Autodesk Inventor part; units mm, degrees
ref_plane "Work Plane2" through (26.9102, -85.3653, -23.8679) normal (0, 0, -1) x (0, 1, 0)
ref_plane "YZ Plane" through (0, 0, 0) normal (1, 0, 0) x (0, 1, 0)
ref_plane "XZ Plane" through (0, 0, 0) normal (0, 1, 0) x (-1, 0, 0)
ref_plane "Work Plane1" through (29.8677, -69.0107, 8.183) normal (0, 0, -1) x (-1, 0, 0)
sketch "Sketch1" plane through (29.8677, -69.0107, 8.183) normal (0, 0, -1) x (-1, 0, 0)
  line L0 (2.603, -2) -> (2.603, -17.5)
  line L1 (2.603, -17.5) -> (-10.897, -17.5)
  line L2 (-10.897, -17.5) -> (-10.897, -2)
  line L3 (-10.897, -2) -> (2.603, -2)
  circle A0 centre (6.603, -27.5) radius 1
  circle A1 centre (-13.897, -21) radius 1
  circle A2 centre (1.603, 0.5) radius 1
  arc A3 (9.303, -26.8555) -> (8.303, -25.8555) centre (8.303, -26.8555) ccw
  line L4 (8.303, -25.8555) -> (5.5653, -25.8555)
  arc A4 (4.5653, -24.8555) -> (5.5653, -25.8555) centre (5.5653, -24.8555) ccw
  line L5 (4.5653, -24.8555) -> (4.5653, 2)
  arc A5 (4.5653, 2) -> (3.5653, 3) centre (3.5653, 2) ccw
  line L6 (3.5653, 3) -> (1, 3)
  arc A6 (1, 3) -> (0, 2) centre (1, 2) ccw
  line L7 (0, 2) -> (0, 1)
  arc A7 (-1, 0) -> (0, 1) centre (-1, 1) ccw
  line L8 (-1, 0) -> (-12.5347, 0)
  line L9 (-12.5347, 0) -> (-12.5347, -18.4723)
  arc A8 (-13.5347, -19.4723) -> (-12.5347, -18.4723) centre (-13.5347, -18.4723) ccw
  line L10 (-13.5347, -19.4723) -> (-15.397, -19.4723)
  arc A9 (-15.397, -19.4723) -> (-16.397, -20.4723) centre (-15.397, -20.4723) ccw
  line L11 (-16.397, -20.4723) -> (-16.397, -30)
  line L12 (-16.397, -30) -> (9.303, -30)
  line L13 (9.303, -30) -> (9.303, -26.8555)
  line L14 (-17.397, 11.7453) -> (12.5653, 11.7453)
  line L15 (12.5653, 11.7453) -> (12.5653, -32.2547)
  line L16 (12.5653, -32.2547) -> (-17.397, -32.2547)
  line L17 (-17.397, -32.2547) -> (-17.397, 11.7453)
  line L18 (1.2141, -1.4589) -> (-9.519, -1.4589)
  line L19 (-9.519, -1.4589) -> (-9.519, -23.1404)
  line L20 (-9.519, -23.1404) -> (1.2141, -23.1404)
  line L21 (1.2141, -23.1404) -> (1.2141, -1.4589)
  ellipse E0 centre (-3.397, -10.2547) end of major axis (-6.4323, -10.2547) minor radius 3.0277
  point P0 (29.8677, 69.0107)
  dimension "d0" = 8
  dimension "d1" = 1
  dimension "d13" = 22
  dimension "d14" = 22
extrude "Extrusion1" add sketch "Sketch1" along normal blind 5 contours L13 L12 L11 A9 L10 A8 L9 L8 A7 L7 A6 L6 A5 L5 A4 L4 A3 | L14 L15 L16 L17
sketch "Sketch2" plane through (29.8677, -69.0107, 3.183) normal (0, 0, -1) x (-1, 0, 0)
  line L0 (12.5653, 11.7453) -> (-17.397, 11.7453)
  line L1 (-17.397, 11.7453) -> (-17.397, -32.2547)
  line L2 (-17.397, -32.2547) -> (12.5653, -32.2547)
  line L3 (12.5653, -32.2547) -> (12.5653, 11.7453)
  circle A0 centre (6.603, -27.5) radius 1
  circle A1 centre (-13.897, -21) radius 1
  circle A2 centre (1.603, 0.5) radius 1
  line L4 (1.2141, -17.5) -> (1.2141, -23.1404)
  line L5 (1.2141, -23.1404) -> (-9.519, -23.1404)
  line L6 (-9.519, -23.1404) -> (-9.519, -17.5)
  line L7 (-9.519, -17.5) -> (-10.897, -17.5)
  line L8 (-10.897, -17.5) -> (-10.897, -2)
  line L9 (-10.897, -2) -> (-9.519, -2)
  line L10 (-9.519, -2) -> (-9.519, -1.4589)
  line L11 (-9.519, -1.4589) -> (1.2141, -1.4589)
  line L12 (1.2141, -1.4589) -> (1.2141, -2)
  line L13 (1.2141, -2) -> (2.603, -2)
  line L14 (2.603, -2) -> (2.603, -17.5)
  line L15 (2.603, -17.5) -> (1.2141, -17.5)
  line L16 (-17.397, 11.7453) -> (12.5653, 11.7453)
  line L17 (12.5653, -32.2547) -> (-17.397, -32.2547)
  line L18 (12.5653, 11.7453) -> (6.5653, 11.7453)
  line L19 (6.5653, 11.7453) -> (6.5653, -32.2547)
  line L20 (6.5653, -32.2547) -> (12.5653, -32.2547)
  line L21 (12.5653, -32.2547) -> (12.5653, 11.7453)
  point P0 (29.8677, 69.0107)
  dimension "d6" = 6
extrude "Extrusion2" add sketch "Sketch2" along normal blind 32 contours L3 L2 L19 A0 L0 | A0 L19 picked at (6.9324, -27.235)
sketch "Sketch3" plane through (29.8677, -69.0107, -28.817) normal (0, 0, -1) x (-1, 0, 0)
  circle A0 centre (-3.397, -10) radius 4.445
  circle A1 centre (-3.397, -10) radius 4.645
  line L0 (12.5653, 11.7453) -> (12.5653, -32.2547)
  line L1 (12.5653, -32.2547) -> (12.5653, 11.7453)
  line L2 (12.5653, 11.7453) -> (6.5653, 11.7453)
  line L3 (6.5653, 11.7453) -> (6.5653, -32.2547)
  line L4 (6.5653, -32.2547) -> (12.5653, -32.2547)
  line L5 (12.5653, -32.2547) -> (12.5653, 11.7453)
  line L6 (6.5653, 11.7453) -> (-17.397, 11.7453)
  line L7 (-9.2429, -0.682) -> (6.5653, 11.7453)
  line L8 (-9.5834, -19.0955) -> (6.5653, -32.2547)
  line L9 (6.5653, 11.7453) -> (6.5653, -5.3362)
  line L10 (6.5653, -14.6638) -> (6.5653, -32.2547)
  arc A2 (-9.2429, -0.682) -> (-9.5834, -19.0955) centre (-3.397, -10) ccw
  arc A3 (6.5653, -14.6638) -> (6.5653, -5.3362) centre (-3.397, -10) ccw
  point P0 (29.8677, 69.0107)
  dimension "d9" = 0.2
ref_plane "Work Plane2" through (26.9102, -85.3653, -23.8679) normal (0, 0, -1) x (0, 1, 0)
extrude "Extrusion3" add sketch "Sketch3" against normal up to surface (4.9491 mm away) contours L0 L4 L3 A3 L2 | L3 L8 A2 L7 | A3 L3
ref_plane "Work Plane3" through (29.8677, -69.0107, -2.817) normal (0, 0, -1) x (-1, 0, 0)
sketch "Sketch4" plane through (29.8677, -69.0107, -2.817) normal (0, 0, -1) x (-1, 0, 0)
  circle A0 centre (-3.397, -10) radius 6.35
  line L0 (6.5653, -32.2547) -> (6.5653, 11.7453)
  line L1 (6.5653, -32.2547) -> (-4.8237, -20.0055)
  line L2 (-4.8237, -20.0055) -> (-4.8237, -16.1877)
  line L3 (12.5653, -32.2547) -> (-17.397, -32.2547)
  line L4 (6.5653, 11.7453) -> (-4.8237, -0.7453)
  line L5 (-4.8237, -0.7453) -> (-4.8237, -3.8123)
  point P0 (29.8677, 69.0107)
extrude "Extrusion4" add sketch "Sketch4" along normal blind 10 contours A0 L5 L4 L0 L1 L2
sketch "Sketch5" plane through (23.3024, -101.2655, -23.8679) normal (1, 0, 0) x (0, 0, -1)
  line L0 (-21.0509, 0) -> (-21.0509, 44)
  line L1 (-27.0509, 44) -> (-21.0509, 44)
  line L2 (-27.0509, 0) -> (-27.0509, 3.7554)
  line L3 (-27.0509, 0) -> (-21.0509, 0)
  line L4 (-11.0509, 44) -> (-11.0509, 0)
  line L5 (-11.0509, 0) -> (0, 0)
  line L6 (-11.0509, 44) -> (0, 44)
  line L7 (-5.3231, 32.8665) -> (-5.3231, 11.3659)
  line L8 (-5.3231, 11.3659) -> (-23.9432, 22.1162)
  line L9 (-23.9432, 22.1162) -> (-5.3231, 32.8665)
  circle A0 centre (-23.9432, 22.1162) radius 3
  circle A1 centre (-5.3231, 32.8665) radius 3
  circle A2 centre (-5.3231, 11.3659) radius 3
  line L10 (-27.0509, 0) -> (-21.0509, 0)
  line L11 (-27.0509, 44) -> (-21.0509, 44)
  line L12 (-21.0509, 0) -> (-21.0509, 44)
  line L13 (-27.0509, 5.754) -> (-27.0509, 44)
  line L14 (-27.0509, 5.754) -> (-27.0509, 3.7554)
  line L15 (-27.0509, 0) -> (-27.0509, 3.7554)
  line L16 (-27.0509, 5.754) -> (-27.0509, 44)
  line L17 (-27.0509, 5.754) -> (-27.0509, 3.7554)
  line L18 (0, 0) -> (0, 44)
  point P0 (-23.8679, 101.2655)
  point P1 (-11.5298, 22.1162)
  dimension "d18" = 0
  dimension "d19" = 6
  dimension "d20" = 6
  dimension "d21" = 6
extrude "Extrusion5" cut sketch "Sketch5" against normal blind 10 contours A0 L8 L9 L0 | L0 A0 | A0 L9 L8 | A2 L7 L8 | L8 L7 A2 | A1 L7 L9 | L9 L7 A1
properties part number "30_cellSTORM_fiberbase_base_v3"
Source: CAD feature listing. Evaluate the final solid. Frame: model axes, mm. A direction names the side the tool comes from. Round coordinates to 2 decimals unless told otherwise and drop trailing zeros. Loops run counter-clockwise (first coordinate to the right, second up) from the corner with the lowest first, then second, coordinate; pieces in that order, holes last. Notation, with made-up numbers: (80, 55) - (132, 55) arc R17 ccw to (132, 87) - close; hole circle Ø1 at (30, 78.25). An arc over 180 degrees is marked (long way). Use CSV: the item, a comma, the result in double quotes.
Q1. Section query D-D, the plane y = -84.5. Output: boundary loops of the cut face in (x, z), then the cut area to 3 significant figures.
Reported:
outline,"(17.3, -28.82) - (42.8, -28.82) - (42.8, -23.87) - (23.3, -23.87) - (23.3, -12.82) - (30.07, -12.82) - (30.07, -2.82) - (23.3, -2.82) - (23.3, 3.18) - (27.26, 3.18) - (27.26, 8.18) - (17.3, 8.18) - close; (40.76, 3.18) - (47.26, 3.18) - (47.26, 8.18) - (40.76, 8.18) - close"
area,"438 mm^2"
Q2. Reachability of faces 1 (the flat face through (31.49, -94.594, -26.377)), 2 (the flat face through (28.654, -89, 6)), 3 (the flat face through (34.691, -87, -8)), 4 (the cylindrical face through (44.26, -78.65, -26.38)), 5 (the flat face through (26.5, -79, -2.817)) from +Z, -Z, +X, -X, +Y, -Y: full face, straight path, thin tool, end or side. Return the list, or none.
Reported:
face 1,"-Z, +X, -Y"
face 2,"+Z"
face 3,"+Z, +X, +Y, -Y"
face 4,"-Z, +X"
face 5,"+X, +Y, -Y"
Q3. Section query C-C, the plane x = 31.5. Output: boundary loops of the cut face in (y, z), then the cut area to 3 significant figures.
Reported:
outline,"(-101.27, 3.18) - (-92.15, 3.18) - (-92.15, 8.18) - (-101.27, 8.18) - close; (-94.59, -28.82) - (-83.31, -28.82) - (-83.31, -23.87) - (-94.59, -23.87) - close; (-92.45, -12.82) - (-85.11, -12.82) - (-85.11, -2.82) - (-92.45, -2.82) - close; (-74.71, -28.82) - (-63.71, -28.82) - (-63.71, -23.87) - (-74.71, -23.87) - close; (-72.91, -12.82) - (-66.26, -12.82) - (-66.26, -2.82) - (-72.91, -2.82) - close; (-70.47, 3.18) - (-57.27, 3.18) - (-57.27, 8.18) - (-70.47, 8.18) - close"
area,"362 mm^2"
Q4. Section query A-A, the plane z = 6. Output: boundary loops of the cut face in (x, y).
Reported:
outline,"(17.3, -101.27) - (47.26, -101.27) - (47.26, -57.27) - (17.3, -57.27) - close; hole circle Ø2 at (23.26, -96.51); hole (27.26, -86.51) - (28.65, -86.51) - (28.65, -92.15) - (39.39, -92.15) - (39.39, -86.51) - (40.76, -86.51) - (40.76, -71.01) - (39.39, -71.01) - (39.39, -70.47) - (28.65, -70.47) - (28.65, -71.01) - (27.26, -71.01) - close; hole circle Ø2 at (28.26, -68.51); hole circle Ø2 at (43.76, -90.01)"
Q5. Section query B-B, the plane x = 20.5. Output: boundary loops of the cut face in (y, z), then the cut area to 3 significant figures.
Reported:
outline,"(-101.27, -28.82) - (-57.27, -28.82) - (-57.27, 8.18) - (-101.27, 8.18) - close; hole circle Ø6 at (-89.9, -18.54); hole circle Ø6 at (-79.15, 0.08); hole circle Ø6 at (-68.4, -18.54)"
area,"1,540 mm^2"
Q6. Pin query (flat end, axial travel): pin 1 Ø8 at (x, y) = (41.5, -92) entering from -Z; pin 2 Ø6.5 at (y, z) = (-88, -0.5) entering from +X. Return the tip coordinate at first contact, or that it passes through.
Reported:
pin 1,"z = 3.18"
pin 2,"x = 34.69"
Q7. Mould query, pull axis Z, two halves, no side actions, for faces 6 (the flat face through (23, -96, 3.183)), 7 (the flat face through (22, -57.265, -2)), 8 (the flat face through (23.302, -79, -18)). Classes: pulls with the +Z half, pulls with the -Z half, needs draft (parallel to the pull), parting line crosses it, or undercut.
Reported:
face 6,"pulls with the +Z half"
face 7,"needs draft"
face 8,"undercut"
Q8. Ray query, line 1 along Z through (x, y) = (27, -94); line 2 along X through (y, z) = (-76, 4); line 3 along Y through (x, z) = (27.5, 6.5). Return the intervals inside material, ascending.
Reported:
line 1,"-28.82 to -23.87, -12.82 to -2.82, 3.18 to 8.18"
line 2,"17.3 to 27.26, 40.76 to 47.26"
line 3,"-101.27 to -86.51, -71.01 to -69.16, -67.87 to -57.27"
